from build123d import *

# Parameters (mm, degrees)
BOSS_EXTRUDE1_DEPTH = 5
SKETCH2_R           = 15
BOSS_EXTRUDE2_DEPTH = 10


with BuildPart() as part:
    # Sketch1 → Boss-Extrude1 (new, symmetric)
    with BuildSketch(Plane(origin=(0, 0, 0), x_dir=(1, 0, 0), z_dir=(0, 1, 0))):
        with BuildLine():
            Line((65, -20), (-65, -20))
            ThreePointArc((-65, -20), (-85, 0), (-65, 20))
            Line((-65, 20), (65, 20))
            Line((65, 20), (65, -20))
        make_face()
        with BuildLine():
            Line((-65, 10), (-25, 10))
            ThreePointArc((-25, 10), (-15, 0), (-25, -10))
            Line((-25, -10), (-65, -10))
            ThreePointArc((-65, -10), (-75, 0), (-65, 10))
        make_face(mode=Mode.SUBTRACT)
    extrude(amount=BOSS_EXTRUDE1_DEPTH, both=True)

    # Sketch2 → Boss-Extrude2 (add)
    with BuildSketch(Plane.XY.offset(20)):
        with BuildLine():
            Line((65, 5), (15, 5))
            Line((15, 5), (15, 35))
            ThreePointArc((15, 35), (40, 60), (65, 35))
            Line((65, 35), (65, 5))
        make_face()
        with Locations((40, 35)):
            Circle(SKETCH2_R, mode=Mode.SUBTRACT)
    boss_extrude2 = extrude(amount=-BOSS_EXTRUDE2_DEPTH)

    # Mirror1: Boss-Extrude2 across plane
    add(boss_extrude2.mirror(Plane.XY))


solid = part.part
The model under review builds one solid part; all positions refer to its coordinate system, in mm. A direction names the side the tool comes from. Round coordinates to 2 decimals unless told otherwise and drop trailing zeros. Order: outer loops, then holes, each group sorted by start corner. A loop starts at its lowest first (then second) coordinate and runs counter-clockwise, first axis right, second up. Notation, with made-up numbers: (23, 10) -> (57, 10) arc R7 cw to (57, 22) -> close; hole circle Ø3 at (-30, 77). An arc over 180 degrees is marked (long way). Use CSV: the item, a comma, the result in double quotes. Start each with the question number.
(1) Consider section A-A on y = 26. Write out the cut boundary in (x, z).
(2) Consider section B-B on x = -36.5. Write out the cut boundary in (y, z), and give its area (3 significant figures).
(3) Wall thickness on probe 1 along Y at (x, z) = (40, 16); probe 2 along Z at (x, y) = (29, 12); probe 3 along Y at (x, z) = (7, -7): over which ranges is each line inside the solid? List them lowest first. Write a range as from..to.
(4) Mouldability with a two-part tool opening along Z and no side actions: class faces 1 (the face through (39.45, 59.994, -15.07)), 2 (the face through (-45, 0, 10)), 3 (the face through (30, 21, -20)) as pulls with the +Z half, pulls with the -Z half, needs draft (parallel to the pull), parting line crosses it, or undercut.
(5) Consider section D-D on x = 40. Write out the cut boundary in (y, z).
(6) Insertion check: pin 1 (8 mm diameter, centred on y = 37.5, z = 14.5, fed in from -X); pin 2 (6 mm diameter, centred on x = 44, y = 46, fed in from +Z); pin 3 (2 mm diameter, centred on x = 32, z = -9.5, fed in from +Y). Each pin has a flat end and moves straight along its axis. Give the tip position at first contact, or say it passes through.
(7) Consider section C-C on z = 0. Write out the cut boundary in (x, y), and give its area (3 significant figures).
(8) Tool access review of faces 4 (the face through (15, 20, -15)), 5 (the face through (-45, 0, -10)), 6 (the face through (34.8, 20.7, 10)): name each direction out of +Z, -Z, +X, -X, +Y, -Y from which nothing blocks a thin tool from reaching the whole face with its end or side.
Responses:
1,outline,"(15, -20) -> (28, -20) -> (28, -10) -> (15, -10) -> close; (15, 10) -> (28, 10) -> (28, 20) -> (15, 20) -> close; (52, -20) -> (65, -20) -> (65, -10) -> (52, -10) -> close; (52, 10) -> (65, 10) -> (65, 20) -> (52, 20) -> close"
2,outline,"(-5, -20) -> (5, -20) -> (5, -10) -> (-5, -10) -> close; (-5, 10) -> (5, 10) -> (5, 20) -> (-5, 20) -> close"
2,area,"200 mm²"
3,probe 1,"-5..20, 50..60"
3,probe 2,"-20..-10, 10..20"
3,probe 3,"-5..5"
4,face 1,"needs draft"
4,face 2,"undercut"
4,face 3,"pulls with the -Z half"
5,outline,"(-5, -20) -> (20, -20) -> (20, -10) -> (5, -10) -> (5, 10) -> (20, 10) -> (20, 20) -> (-5, 20) -> close; (50, -20) -> (60, -20) -> (60, -10) -> (50, -10) -> close; (50, 10) -> (60, 10) -> (60, 20) -> (50, 20) -> close"
6,pin 1,"x = 15"
6,pin 2,"through"
6,pin 3,"y = 58.96"
7,outline,"(-85, -5) -> (-75, -5) -> (-75, 5) -> (-85, 5) -> close; (-15, -5) -> (65, -5) -> (65, 5) -> (-15, 5) -> close"
7,area,"900 mm²"
8,face 4,"+Z, -Z, -X, +Y"
8,face 5,"+Y, -Y"
8,face 6,"+X, -X, +Y"
